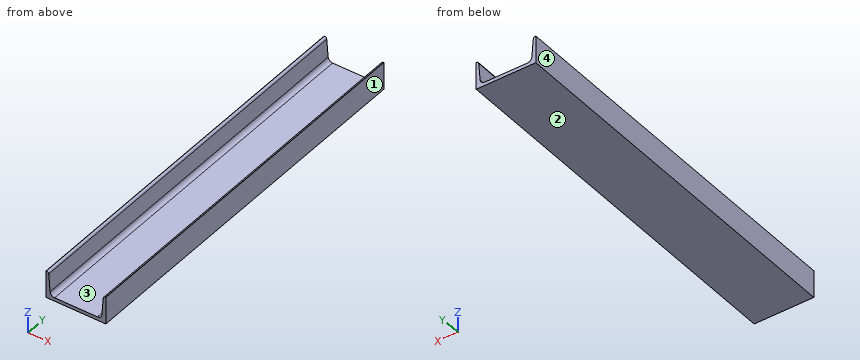
```python
from build123d import *

# Parameters (mm, degrees)
F1_DEPTH = 770


with BuildPart() as f1:
    # F0 (on Front) → F1 (new body)
    with BuildSketch(Plane.XZ):
        with BuildLine():
            Line((0.645623, 55), (0, 55))
            Line((0, 55), (0, 0))
            Line((0, 0), (120, 0))
            Line((120, 0), (120, 55))
            Line((120, 55), (119.354377, 55))
            ThreePointArc((119.354377, 55), (116.301906, 53.806421), (114.868708, 50.858854))
            Line((114.868708, 50.858854), (112.022583, 15.282293))
            ThreePointArc((112.022583, 15.282293), (109.156188, 9.387158), (103.051246, 7))
            Line((103.051246, 7), (16.948754, 7))
            ThreePointArc((16.948754, 7), (10.843812, 9.387158), (7.977417, 15.282293))
            Line((7.977417, 15.282293), (5.131292, 50.858854))
            ThreePointArc((5.131292, 50.858854), (3.698094, 53.806421), (0.645623, 55))
        make_face()
    extrude(amount=F1_DEPTH)


solid = f1.part
```
CAD build for the part. Positions are in the model's coordinates, mm. Face numbers are marked on the shaded views. Coordinates: 2 decimals unless noted, no trailing zeros. Order: outer loops, then holes, each group sorted by start corner. A loop starts at its lowest first (then second) coordinate and runs counter-clockwise, first axis right, second up. Notation, with made-up numbers: M -12.75,-15 L 3.25,-15 A18 ccw 3.25,1 Z; hole C -31.75,46.25 d5. An arc over 180 degrees is marked long. Write each question's results on one line, items separated by ' | '. Start each with the question number.
Q1. Cut at B-B (y = -187). List the corners of the cut face in (x, z).
Q2. Flat gauge pin, fed straight in: P1, Ø12, axis at x = 86, y = -478, coming from the +Z side. Where does the tip first touch, or does it go through?
Q3. Pull direction X, two halves, no side cores. Call the marked faces 1, 2, 3 and 4: +X half, -X half, draft (parallel to the pull), parting line (faces both ways), or undercut.
Q4. Cut at A-A (z = 41). List the corners of the cut face in (x, y), then the cut area to 3 significant figures.
Q5. Drill centre lines: probe 1 along X at (y, z) = (-41, 16.5); probe 2 along Z at (x, y) = (85, -540); probe 3 along X at (y, z) = (-558, 50.5). Where is each one in solid material? Low to high. Write a range as from..to.
Q6. Cut at C-C (x = 82). List the corners of the cut face in (y, z), then the cut area to 3 significant figures.
Found:
1) outline: M 0,0 L 120,0 L 120,55 L 119.35,55 A4.5 ccw 114.87,50.86 L 112.02,15.28 A9 cw 103.05,7 L 16.95,7 A9 cw 7.98,15.28 L 5.13,50.86 A4.5 ccw 0.65,55 L 0,55 Z
2) P1: z = 7
3) face 1: +X half | face 2: draft | face 3: undercut | face 4: -X half
4) outline: M 0,-770 L 5.92,-770 L 5.92,0 L 0,0 Z; M 114.08,-770 L 120,-770 L 120,0 L 114.08,0 Z | area: 9,120 mm²
5) probe 1: 0..7.88, 112.12..120 | probe 2: 0..7 | probe 3: 0..5.16, 114.84..120
6) outline: M -770,0 L 0,0 L 0,7 L -770,7 Z | area: 5,390 mm²
